```python
from build123d import *

# Parameters (mm, degrees)
SKETCH009_W          = 16
SKETCH009_H          = 25.5
PAD003_DEPTH         = 1.5
PAD003_DEPTH_BACK    = 18.5
POCKET006_DEPTH      = 12.751
POCKET006_DEPTH_BACK = 12.751
SKETCH010_R          = 2.25
PAD004_DEPTH         = 2.9
SKETCH011_R          = 2.25
PAD005_DEPTH         = 2.9
POCKET002_DEPTH      = 11.35
POCKET003_DEPTH      = 11.35
SKETCH015_R          = 2.2
POCKET004_DEPTH      = 26.501032
SKETCH016_R          = 3.75
POCKET005_DEPTH      = 23.501032
SKETCH017_W          = 6.75
SKETCH017_H          = 5.8
PAD006_DEPTH         = 5
FILLET001_R          = 1


with BuildPart() as part:
    # Sketch009 → Pad003 (new body, two sides)
    with BuildSketch(Plane.XY) as pad003_sk:
        Rectangle(SKETCH009_W, SKETCH009_H)
    extrude(amount=PAD003_DEPTH)
    extrude(pad003_sk.sketch, amount=-PAD003_DEPTH_BACK)

    # Sketch018 → Pocket006 (cut, two sides)
    with BuildSketch(Plane.XZ) as pocket006_sk:
        Polygon((-6, -18.5), (8, 0), (8, -18.5), align=None)
    extrude(amount=-POCKET006_DEPTH, mode=Mode.SUBTRACT)
    extrude(pocket006_sk.sketch, amount=POCKET006_DEPTH_BACK, mode=Mode.SUBTRACT)

    # Sketch010 → Pad004 (join)
    with BuildSketch(Plane.XZ.offset(12.75)):
        with BuildLine():
            ThreePointArc((12.25, 0), (18.500032, 6.25), (12.25, 12.5))
            Line((12.25, 12.5), (0.660254, 12.5))
            Line((0.660254, 12.5), (-8, 7.5))
            Line((-8, 7.5), (-8, 0))
            Line((-8, 0), (12.25, 0))
        make_face()
        with Locations((12.25, 6.25)):
            Circle(SKETCH010_R, mode=Mode.SUBTRACT)
    extrude(amount=-PAD004_DEPTH)

    # Sketch011 → Pad005 (join)
    with BuildSketch(Plane.XZ.offset(-12.75)):
        with BuildLine():
            Line((12.25, 0), (-8, 0))
            Line((-8, 0), (-8, 7.5))
            Line((-8, 7.5), (0.660254, 12.5))
            Line((0.660254, 12.5), (12.25, 12.5))
            ThreePointArc((12.25, 0), (18.500019, 6.25), (12.25, 12.5))
        make_face()
        with Locations((12.25, 6.25)):
            Circle(SKETCH011_R, mode=Mode.SUBTRACT)
    extrude(amount=PAD005_DEPTH)

    # Sketch012 → Pocket002 (cut)
    with BuildSketch(Plane.XZ.offset(11.35)):
        with BuildLine():
            Line((18.6, 12.5), (18.6, 0))
            Line((8, 0), (18.6, 0))
            Line((8, 1.005956), (8, 0))
            ThreePointArc((6.50892, 9.8), (5.594985, 5.121605), (8, 1.005956))
            Line((6.50892, 9.8), (11.5, 9.8))
            Line((11.5, 9.8), (11.5, 12.5))
            Line((11.5, 12.5), (18.6, 12.5))
        make_face()
    extrude(amount=-POCKET002_DEPTH, mode=Mode.SUBTRACT)

    # Sketch013 → Pocket003 (cut)
    with BuildSketch(Plane.XZ.offset(-11.35)):
        with BuildLine():
            Line((18.6, 12.5), (18.6, 0))
            Line((8, 0), (18.6, 0))
            Line((8, 1.005956), (8, 0))
            ThreePointArc((6.50892, 9.8), (5.594985, 5.121605), (8, 1.005956))
            Line((6.50892, 9.8), (11.5, 9.8))
            Line((11.5, 9.8), (11.5, 12.5))
            Line((11.5, 12.5), (18.6, 12.5))
        make_face()
    extrude(amount=POCKET003_DEPTH, mode=Mode.SUBTRACT)

    # Sketch015 (on DatumPlane) → Pocket004 (cut, through all)
    with BuildSketch(Plane(origin=(-8, 12.75, 0), x_dir=(0, -1, 0), z_dir=(-1, 0, 0))):
        with Locations((12.75, -8.5)):
            Circle(SKETCH015_R)
    extrude(amount=-POCKET004_DEPTH, mode=Mode.SUBTRACT)

    # Sketch016 (on DatumPlane) → Pocket005 (cut, through all)
    with BuildSketch(Plane(origin=(-5, 12.75, 0), x_dir=(0, -1, 0), z_dir=(-1, 0, 0))):
        with Locations((12.75, -8.5)):
            Circle(SKETCH016_R)
    extrude(amount=-POCKET005_DEPTH, mode=Mode.SUBTRACT)

    # Sketch017 (on DatumPlane) → Pad006 (join)
    with BuildSketch(Plane(origin=(-8, 12.75, 0), x_dir=(0, -1, 0), z_dir=(-1, 0, 0))):
        with Locations((3.375, -8.5)):
            Rectangle(SKETCH017_W, SKETCH017_H)
        with Locations((22.125, -8.5)):
            Rectangle(SKETCH017_W, SKETCH017_H)
    extrude(amount=PAD006_DEPTH)

    # Fillet001
    fillet001_edges = [part.edges().sort_by_distance(p)[0] for p in [
        (1, -12.75, -9.25),
        (1, 12.75, -9.25),
        (-7, 12.75, -18.5),
        (-6, 0, -18.5),
        (-7, -12.75, -18.5),
        (-0.272916, -9.85, 1.5),
        (-0.272916, 9.85, 1.5),
    ]]
    fillet(fillet001_edges, radius=FILLET001_R)


solid = part.part
```
Verification items for the finished model (mm, model axes). A direction names the side the tool comes from. Give positions to 0.01 mm unless a question says otherwise; leave off trailing zeros. Order: outer loops, then holes, each group sorted by start corner. A loop starts at its lowest first (then second) coordinate and runs counter-clockwise, first axis right, second up. Notation, with made-up numbers: (50.5, 2.5) - (94.5, 2.5) arc R25 cw to (94.5, 15.5) - close; hole circle Ø1 at (28, -16). An arc over 180 degrees is marked (long way). Answer as CSV lines item,"result". Start each with the question number.
Item 1: Section check D-D, the plane y = -5. Record the boundary of the cut face in (x, z), plus the area to 3 significant figures.
Item 2: Gauge pin test, flat ends, axial feed: pin 1 (6 mm diameter, centred on y = -1.5, z = -8, fed in from +X); pin 2 (4 mm diameter, centred on x = -10.5, y = 9.5, fed in from +Z); pin 3 (0.8 mm diameter, centred on y = 2, z = 0.5, fed in from +X); pin 4 (3.5 mm diameter, centred on x = 12.25, z = 6.25, fed in from +Y). Record the tip position at first contact, or that the pin passes through.
Item 3: Section check A-A, the plane z = 6.25. Record the boundary of the cut face in (x, y), plus the area to 3 significant figures.
Item 4: Mould release check, pull along Y, two halves, no side actions. Record for faces 5 (the face through (6, 11, 12.5)), 6 (the face through (-7.238, 12.465, -18.199)), 7 (the face through (-1, -9.85, 8)): released by +Y, released by -Y, zero draft, split by the parting line, or undercut.
Item 5: Section check C-C, the plane y = 0. Record the boundary of the cut face in (x, z).
Item 6: Material ranges on L1, parallel to Y at x = 17, z = 7; L2, parallel to Y at x = -1, z = -8.5; L3, parallel to Z at x = 12.25, y = 11.7, recorded low to high.
Item 7: Section check B-B, the plane x = -10.5. Record the boundary of the cut face in (y, z).
Item 8: Access from +Z, -Z, +X, -X, +Y, -Y to the whole of each face (thin tool, end or side, straight path). Record for faces 1 (the face through (-10, -6, -9)), 2 (the face through (0, 0, 1.5)), 3 (the face through (-1.408, 0.488, -4.782)), 4 (the face through (11.5, -11, 11)).
Filled in:
1,outline,"(-8, -18.5) - (-6.5, -18.5) arc R1 ccw to (-5.7, -18.1) - (8, 0) - (8, 1.01) arc R6.75 cw to (7.45, 1.5) - (-8, 1.5) - close"
1,area,"190 mm^2"
2,pin 1,"x = 4.22"
2,pin 2,"z = -5.6"
2,pin 3,"x = 8"
2,pin 4,"through"
3,outline,"(-8, -12.75) - (10, -12.75) - (10, -11.35) - (5.5, -11.35) - (5.5, -9.85) - (-8, -9.85) - close; (-8, 9.85) - (5.5, 9.85) - (5.5, 11.35) - (10, 11.35) - (10, 12.75) - (-8, 12.75) - close; (14.5, -12.75) - (18.5, -12.75) - (18.5, -11.35) - (14.5, -11.35) - close; (14.5, 11.35) - (18.5, 11.35) - (18.5, 12.75) - (14.5, 12.75) - close"
3,area,"102 mm^2"
4,face 5,"zero draft"
4,face 6,"released by +Y"
4,face 7,"undercut"
5,outline,"(-8, -18.5) - (-6.5, -18.5) arc R1 ccw to (-5.7, -18.1) - (-1.27, -12.25) - (-5, -12.25) - (-5, -10.7) - (-8, -10.7) - close; (-8, -6.3) - (-5, -6.3) - (-5, -4.75) - (4.41, -4.75) - (8, 0) - (8, 1.01) arc R6.75 cw to (7.45, 1.5) - (-8, 1.5) - close"
6,L1,"-12.75 to -11.35, 11.35 to 12.75"
6,L2,"-12.75 to -3.75, 3.75 to 12.75"
6,L3,"0 to 4, 8.5 to 12.5"
7,outline,"(-12.75, -11.4) - (-6, -11.4) - (-6, -5.6) - (-12.75, -5.6) - close; (6, -11.4) - (12.75, -11.4) - (12.75, -5.6) - (6, -5.6) - close"
8,face 1,"+Z, -Z, -X"
8,face 2,"+Z, +X, -X"
8,face 3,"+X"
8,face 4,"+Z, -Z, +X"
